The listing builds one solid part. Answer for the finished solid, in the listing's coordinates (mm). A direction names the side the tool comes from. Coordinates: 2 decimals unless noted, no trailing zeros. Order: outer loops, then holes, each group sorted by start corner. A loop starts at its lowest first (then second) coordinate and runs counter-clockwise, first axis right, second up. Notation, with made-up numbers: (1, -34.5) -> (9, -34.5) arc R15 ccw to (9, -12.5) -> close; hole circle Ø3 at (-15.5, -13). An arc over 180 degrees is marked (long way). Return JSON: item names as keys, results as strings.
from build123d import *

# Parameters (mm, degrees)
SKETCH1_R           = 5
BOSS_EXTRUDE1_DEPTH = 3.175
SKETCH2_R           = 6
CUT_EXTRUDE1_DEPTH  = 4.35
CUT_EXTRUDE2_DEPTH  = 1.35
CHAMFER2_SIZE       = 1.5
SKETCH8_R           = 12
SKETCH8_R_2         = 7.5
CUT_EXTRUDE3_DEPTH  = 0.75


with BuildPart() as part:
    # Sketch1 → Boss-Extrude1 (new, symmetric)
    with BuildSketch(Plane(origin=(0, 0, 0), x_dir=(0, 0, -1), z_dir=(1, 0, 0))):
        with BuildLine():
            Line((-10, 35), (10, 35))
            Line((10, 35), (10, 9.797958971))
            ThreePointArc((10, 9.797958971), (0, -14), (-10, 9.797958971))
            Line((-10, 9.797958971), (-10, 35))
        make_face()
        Circle(SKETCH1_R, mode=Mode.SUBTRACT)
    extrude(amount=BOSS_EXTRUDE1_DEPTH, both=True)

    # Sketch2 → Cut-Extrude1 (cut)
    with BuildSketch(Plane.ZY.offset(3.175)):
        Circle(SKETCH2_R)
    extrude(amount=-CUT_EXTRUDE1_DEPTH, mode=Mode.SUBTRACT)

    # Sketch4 → Cut-Extrude2 (cut)
    with BuildSketch(Plane.ZY.offset(-3.175)):
        with BuildLine():
            Line((-16.06497938, 41.777700925), (20.751052424, 41.777700925))
            Line((20.751052424, 41.777700925), (18.684504783, 1.284491351))
            Line((18.684504783, 1.284491351), (13.967034386, 0.960182519))
            ThreePointArc((13.967034386, 0.960182519), (0, 14), (-13.967034386, 0.960182519))
            Line((-13.967034386, 0.960182519), (-15.162675902, -1.531420388))
            Line((-15.162675902, -1.531420388), (-19.899722353, 37.471795214))
            Line((-19.899722353, 37.471795214), (-16.06497938, 41.777700925))
        make_face()
    extrude(amount=CUT_EXTRUDE2_DEPTH, mode=Mode.SUBTRACT)

    # Chamfer2
    # the kernel refuses this chamfer: 1.5 mm, written as the material it adds along each edge
    with BuildSketch(Plane(origin=(1.825, 0, 0), x_dir=(0, 0.4790238441764441, 0.8778018892155689), z_dir=(0, -0.8778018892155689, 0.4790238441764441))) as chamfer2_piece_1_section:
        Polygon((14 + CHAMFER2_SIZE, 0), (14, -CHAMFER2_SIZE), (14, 0), align=None)
    chamfer2_piece_1 = revolve(axis=Axis((1.825, 0, 0), (-1, 0, 0)), revolution_arc=122.756665739, mode=Mode.PRIVATE)
    chamfer2_piece_1 = split(chamfer2_piece_1, bisect_by=Plane(origin=(2.457619264, 14.825045671, 10), z_dir=(0, 0, -1)), keep=Keep.TOP, mode=Mode.PRIVATE)
    chamfer2_piece_1 = split(chamfer2_piece_1, bisect_by=Plane(origin=(3.175, 14.825045671, 0), z_dir=(-1, 0, 0)), keep=Keep.TOP, mode=Mode.PRIVATE)
    chamfer2_piece_1 = split(chamfer2_piece_1, bisect_by=Plane(origin=(2.457619264, 14.825045671, -10), z_dir=(0, 0, 1)), keep=Keep.TOP, mode=Mode.PRIVATE)
    add(chamfer2_piece_1)

    # Sketch8 → Cut-Extrude3 (cut)
    with BuildSketch(Plane.ZY.offset(3.175)):
        Circle(SKETCH8_R)
        Circle(SKETCH8_R_2, mode=Mode.SUBTRACT)
    extrude(amount=-CUT_EXTRUDE3_DEPTH, mode=Mode.SUBTRACT)


solid = part.part
1. The part is cut by section A-A on y = 0. Give the vertices of the cut face in (x, z) (3 decimals), and give its area (4 significant figures).
Answer block:
{"outline": "(-3.175, -14) -> (3.175, -14) -> (3.175, -5) -> (1.175, -5) -> (1.175, -6) -> (-3.175, -6) -> (-3.175, -7.5) -> (-2.425, -7.5) -> (-2.425, -12) -> (-3.175, -12) -> close; (-3.175, 6) -> (1.175, 6) -> (1.175, 5) -> (3.175, 5) -> (3.175, 14) -> (-3.175, 14) -> (-3.175, 12) -> (-2.425, 12) -> (-2.425, 7.5) -> (-3.175, 7.5) -> close", "area": "98.85 mm2"}
2. Each of these flat-tipped pins is pushed along its axis until it touches: pin 1 Ø16 at (y, z) = (25, -0.5) entering from +X (3 decimals); pin 2 Ø8 at (y, z) = (18, -4) entering from +X; pin 3 Ø3 at (x, y) = (-1, 21.5) entering from -Z. Where does it stop, or does it pass through?
Answer block:
{"pin 1": "stops at x = 1.825", "pin 2": "stops at x = 2.89", "pin 3": "stops at z = -10"}
3. The part is cut by section D-D on z = 10.75. Give the vertices of the cut face in (x, y) (3 decimals).
Answer block:
{"outline": "(-3.175, -8.969) -> (3.175, -8.969) -> (3.175, 8.969) -> (-3.175, 8.969) -> (-3.175, 5.333) -> (-2.425, 5.333) -> (-2.425, -5.333) -> (-3.175, -5.333) -> close"}
4. The part is cut by section C-C on x = -0.75. Give the vertices of the cut face in (y, z), and give its area (3 significant figures).
Answer block:
{"outline": "(9.8, -10) -> (35, -10) -> (35, 10) -> (9.8, 10) arc R14 ccw (long way) to start; hole circle Ø12 at (0, 0)", "area": "949 mm2"}
5. For faces 1 (the face through (-1, 23, 10)), 2 (the face through (-2.805, 0.33, -7.493)), 3 (the face through (-1, 23, -10)), determine the directions among +Z, -Z, +X, -X, +Y, -Y from which every point of the face is accessible in a straight line to the end or side of a thin tool.
Answer block:
{"face 1": "+Z, +X, -X, +Y", "face 2": "-X", "face 3": "-Z, +X, -X, +Y"}
6. The part is cut by section B-B on z = 0. Give the vertices of the cut face in (x, y) (3 decimals), and give its area (3 significant figures).
Answer block:
{"outline": "(-3.175, -14) -> (3.175, -14) -> (3.175, -5) -> (1.175, -5) -> (1.175, -6) -> (-3.175, -6) -> (-3.175, -7.5) -> (-2.425, -7.5) -> (-2.425, -12) -> (-3.175, -12) -> close; (-3.175, 6) -> (1.175, 6) -> (1.175, 5) -> (3.175, 5) -> (3.175, 14.15) -> (1.825, 15.5) -> (1.825, 35) -> (-3.175, 35) -> (-3.175, 12) -> (-2.425, 12) -> (-2.425, 7.5) -> (-3.175, 7.5) -> close", "area": "205 mm2"}
7. Determine the mould class of faces 4 (the face through (-2.425, 6, 5)), 5 (the face through (0, -14, 0)), 6 (the face through (-1, 35, 0)), 7 (the face through (1.825, 24, 0)) for opening direction Y: pulls with the +Y half, pulls with the -Y half, needs draft (parallel to the pull), parting line crosses it, or undercut.
Answer block:
{"face 4": "undercut", "face 5": "parting line crosses it", "face 6": "pulls with the +Y half", "face 7": "needs draft"}
8. Consider line 1 (Y direction, x = -2.8, z = 0); line 2 (Y direction, x = -0.7, z = 0); line 3 (Y direction, x = 1.7, z = 0). Determine where each line is inside the solid, lowest interval first. Write a range as from..to.
Answer block:
{"line 1": "y = -14..-12, -7.5..-6, 6..7.5, 12..35", "line 2": "y = -14..-6, 6..35", "line 3": "y = -14..-5, 5..35"}
